Can you work these out from the model? Positions are in its coordinate system, mm. A direction names the side the tool comes from. Round coordinates to 2 decimals unless told otherwise and drop trailing zeros. Loops run counter-clockwise (first coordinate to the right, second up) from the corner with the lowest first, then second, coordinate; pieces in that order, holes last. Notation, with made-up numbers: (-8.75, -18.5) -> (46.25, -18.5) arc R19 cw to (46.25, 17.5) -> close; hole circle Ø9 at (-39, 20.5). An arc over 180 degrees is marked (long way). Write item = value, one per line.
from build123d import *

# Parameters (mm, degrees)
CYLINDER017_R          = 2
CYLINDER017_DEPTH      = 10
CUT011_PLACEMENT_ANGLE = 180
CYLINDER020_R          = 2
CYLINDER020_DEPTH      = 55
CYLINDER021_R          = 1.5
CYLINDER021_DEPTH      = 62
TUBE008_R              = 3.5
TUBE008_R_2            = 1.5
TUBE008_DEPTH          = 3
TUBE009_R              = 3.5
TUBE009_R_2            = 1.5
TUBE009_DEPTH          = 3
CYLINDER016_R          = 2
CYLINDER016_DEPTH      = 10


with BuildPart() as cylinder017:
    # Cylinder017 → Cylinder017 (new body)
    with BuildSketch(Plane.XZ.offset(-8)):
        Circle(CYLINDER017_R)
    extrude(amount=CYLINDER017_DEPTH)


with BuildPart() as rad_b:
    # Sketch005 → Revolve002 (revolve)
    with BuildSketch(Plane.XY):
        Polygon((0, 0), (17, 0), (15, 2), (14.5, 6.2), (12.8, 6.2), (12.5, 5.25), (6.5, 5.25), (4.5, 5.5), (0, 5.5), align=None)
    revolve(axis=Axis((0, 0, 0), (0, -1, 0)))

    # Cut011: cut Cylinder017
    add(cylinder017.part, mode=Mode.SUBTRACT)


with BuildPart() as rad_b_1:
    # Cut011 placement: moved
    add(rad_b.part.moved(Location((0, -40, 0))).rotate(Axis((0, -40, 0), (0, 0, 1)), CUT011_PLACEMENT_ANGLE))


with BuildPart() as cylinder020:
    # Cylinder020 → Cylinder020 (new body)
    with BuildSketch(Plane.XZ.offset(-7.5)):
        Circle(CYLINDER020_R)
    extrude(amount=CYLINDER020_DEPTH)


with BuildPart() as achse_a:
    # Cylinder021 → Cylinder021 (new body)
    with BuildSketch(Plane.XZ.offset(-11)):
        Circle(CYLINDER021_R)
    extrude(amount=CYLINDER021_DEPTH)

    # Fusion031: union Cylinder020
    add(cylinder020.part)


with BuildPart() as obj1:
    # Tube008 → Tube008 (new body)
    with BuildSketch(Plane(origin=(0, 7.5, 0), x_dir=(1, 0, 0), z_dir=(0, 1, 0))):
        Circle(TUBE008_R)
        Circle(TUBE008_R_2, mode=Mode.SUBTRACT)
    extrude(amount=TUBE008_DEPTH)


with BuildPart() as obj2:
    # Tube009 → Tube009 (new body)
    with BuildSketch(Plane(origin=(0, -50.5, 0), x_dir=(1, 0, 0), z_dir=(0, 1, 0))):
        Circle(TUBE009_R)
        Circle(TUBE009_R_2, mode=Mode.SUBTRACT)
    extrude(amount=TUBE009_DEPTH)


with BuildPart() as cylinder016:
    # Cylinder016 → Cylinder016 (new body)
    with BuildSketch(Plane.XZ.offset(-8)):
        Circle(CYLINDER016_R)
    extrude(amount=CYLINDER016_DEPTH)


with BuildPart() as obj3:
    # Sketch005 → Revolve001 (revolve)
    with BuildSketch(Plane.XY):
        Polygon((0, 0), (17, 0), (15, 2), (14.5, 6.2), (12.8, 6.2), (12.5, 5.25), (6.5, 5.25), (4.5, 5.5), (0, 5.5), align=None)
    revolve(axis=Axis((0, 0, 0), (0, -1, 0)))

    # Cut010: cut Cylinder016
    add(cylinder016.part, mode=Mode.SUBTRACT)

    # Fusion078: union Rad-B, Achse-A, obj1, obj2
    add(rad_b_1.part)
    add(achse_a.part)
    add(obj1.part)
    add(obj2.part)


solid = obj3.part
1. For faces 4 (the flat face through (0, 11, 0)), 5 (the cylindrical face through (-1.5, 10.75, 0.07)), 6 (the flat face through (1, 5.5, -2)), 7 (the cylindrical face through (-1.5, -50.75, 0.07)), which set-ups out of +Z, -Z, +X, -X, +Y, -Y let a thin tool reach every point of the face, with its end or its side?
Entries:
face_4 = +Z, -Z, +X, -X, +Y
face_5 = +Y
face_6 = none
face_7 = -Y
2. I'm going to push flat-ended pins straight in: pin 1 (10 mm diameter, centred on x = -4.5, z = -6.5, fed in from -Y); pin 2 (10 mm diameter, centred on x = 6, y = -11, fed in from -Z); pin 3 (2 mm diameter, centred on x = 12, z = 1.5, fed in from +Y). Where does each tip first touch, or does it pass through?
Entries:
pin_1 = -50.5
pin_2 = -1.73
pin_3 = 6.2
3. Suppose I cut it at A-A, the plane y = -13.5. List the corners of the cut face in (x, z) for me, and give its area (3 significant figures).
Entries:
outline = circle Ø4 at (0, 0)
area = 12.6 mm²
4. We'd pull the mould along Z, two halves only. Please class faces 1 (the flat face through (5, 5.25, -5)), 2 (the flat face through (0, 10.5, 2)), 3 (the cylindrical face through (3.233, -49.021, 1.341)): released by +Z, released by -Z, zero draft, split by the parting line, or undercut.
Entries:
face_1 = undercut
face_2 = zero draft
face_3 = split by the parting line
5. I need wall thicknesses on line 1 (Y direction, x = -12, z = -8); line 2 (Y direction, x = -9, z = -3.5); line 3 (X direction, y = 6, z = 8). Which ranges of each line are inside material? Lowest first, please. Write a range as [from, to].
Entries:
line_1 = [-46.2, -40], [0, 6.2]
line_2 = [-45.25, -40], [0, 5.25]
line_3 = [-12.12, -9.91], [9.91, 12.12]
